For this review, take the finished solid that the model builds, in its own axes (mm). Face numbers are marked on the shaded views. Give positions to 0.01 mm unless a question says otherwise; leave off trailing zeros. Write each loop counter-clockwise with the first axis right and the second up, starting at its lowest first coordinate (ties: lowest second). Pieces come first, ordered by that corner, then holes.
1) We need section A-A on y = -4.5. Give the boundary of the cut face in (x, z), and give its area (3 significant figures).
2) Draft analysis for pull direction Y (two halves, no side actions). For the marked faces 1, 2 and 3, state which applies: pulls with the +Y half, pulls with the -Y half, needs draft (parallel to the pull), parting line crosses it, or undercut.
3) For P1, Ø3, axis at x = 36, z = 3, coming from the +Y side, flat-tipped, find the tip position at first contact; note if it passes through.
4) We need section D-D on x = 11. Give the boundary of the cut face in (y, z), and give its area (3 significant figures).
5) Wall thickness on line 1 along X through (y, z) = (-7, 4.4); line 2 along Y through (x, z) = (20, 0.9); line 3 along Y through (x, z) = (44, 3.1): over which ranges is each line inside the solid? List them lowest first.
6) We need section B-B on z = 4.95. Give the boundary of the cut face in (x, y), and give its area (3 significant figures).
7) We need section C-C on y = -36.5. Give the boundary of the cut face in (x, z), and give its area (3 significant figures).
Autodesk Inventor part; units mm, degrees
ref_plane "YZ Plane" through (0, 0, 0) normal (1, 0, 0) x (0, 1, 0)
ref_plane "XZ Plane" through (0, 0, 0) normal (0, 1, 0) x (-1, 0, 0)
ref_plane "XY Plane" through (0, 0, 0) normal (0, 0, 1) x (1, 0, 0)
sketch "Esquisse1" plane through (0, 0, 0) normal (0, 0, 1) x (1, 0, 0)
  line L0 (60, 0) -> (60, -65)
  line L1 (0, 0) -> (0, -6)
  arc A0 (56.6718, -65) -> (60, -65) centre (58.3359, -67.8823) ccw
  line L2 (0, 0) -> (10, 0)
  line L3 (10, 0) -> (10, -6)
  line L4 (10, -6) -> (50, -6)
  line L5 (50, -6) -> (50, 0)
  line L6 (0, 0) -> (10, 0)
  line L7 (50, 0) -> (60, 0)
  line L8 (0, -6) -> (0, -21)
  arc A1 (56.6718, -65) -> (0, -21) centre (1.6431, -77.3802) ccw
  dimension "d0" = 60
  dimension "d1" = 65
  dimension "d2" = 6
  dimension "d5" = 10
  dimension "d6" = 10
  dimension "d8" = 15
extrude "Extrusion1" add sketch "Esquisse1" along normal blind 6
properties part number "roue_libre"
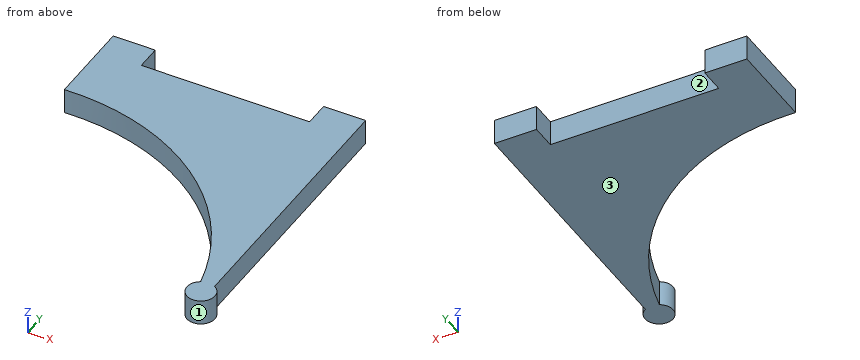
Results list:
1. outline: (0, 0) - (10, 0) - (10, 6) - (0, 6) - close; (50, 0) - (60, 0) - (60, 6) - (50, 6) - close
1. area: 120 mm2
2. face 1: undercut
2. face 2: pulls with the +Y half
2. face 3: needs draft
3. P1: stops at y = -6
4. outline: (-21.76, 0) - (-6, 0) - (-6, 6) - (-21.76, 6) - close
4. area: 94.5 mm2
5. line 1: x = 0 to 60
5. line 2: y = -24.05 to -6
5. line 3: y = -40.13 to -6
6. outline: (0, -21) arc R56.4 cw to (56.67, -65) arc R3.33 ccw (long way) to (60, -65) - (60, 0) - (50, 0) - (50, -6) - (10, -6) - (10, 0) - (0, 0) - close
6. area: 1,820 mm2
7. outline: (40.5, 0) - (60, 0) - (60, 6) - (40.5, 6) - close
7. area: 117 mm2
